For this review, take the finished solid that the model builds, in its own axes (mm). Face numbers are marked on the shaded views. A direction names the side the tool comes from. Round coordinates to 2 decimals unless told otherwise and drop trailing zeros. Write each loop counter-clockwise with the first axis right and the second up, starting at its lowest first coordinate (ties: lowest second). Pieces come first, ordered by that corner, then holes. Notation, with made-up numbers: (-12, -27.5) -> (-5, -27.5) arc R6 ccw to (-5, -23.5) -> close; hole circle Ø7 at (8.5, -27.75). An arc over 180 degrees is marked (long way). Answer in a Markdown table with one row per item.
from build123d import *

# Parameters (mm, degrees)
F0_R           = 14
F1_DEPTH       = 40
F4_D           = 11
F4_CBORE_D     = 18
F4_CBORE_DEPTH = 7.3


with BuildPart() as f1:
    # F0 (on Front) → F1 (new body)
    with BuildSketch(Plane.XZ):
        with BuildLine():
            Line((-31.928091, 15), (-31.928091, 7.7))
            Line((-31.928091, 7.7), (-31.928091, 0))
            Line((-31.928091, 0), (78.071909, 0))
            Line((78.071909, 0), (78.071909, 7.7))
            Line((78.071909, 7.7), (78.071909, 15))
            Line((78.071909, 15), (48.071909, 15))
            Line((48.071909, 15), (48.071909, 27.340618))
            Line((48.071909, 27.340618), (48.071909, 40))
            ThreePointArc((48.071909, 40), (23.071909, 65), (-1.928091, 40))
            Line((-1.928091, 40), (-1.928091, 27.340618))
            Line((-1.928091, 27.340618), (-1.928091, 15))
            Line((-1.928091, 15), (-31.928091, 15))
        make_face()
        with Locations((23.071909, 40)):
            Circle(F0_R, mode=Mode.SUBTRACT)
    extrude(amount=F1_DEPTH)

    # F4 (through all)
    with Locations(Plane.XY.offset(15)):
        with Locations((-16.928091, -20), (63.071909, -20)):
            CounterBoreHole(F4_D / 2, F4_CBORE_D / 2, F4_CBORE_DEPTH)


solid = f1.part
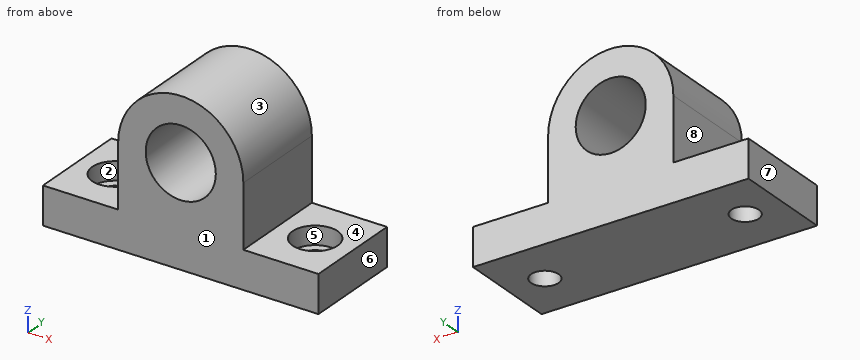
1) Clearance check with flat-ended pins moving along their axes: pin 1 Ø20 at (x, y) = (-16, -16.5) entering from +Z; pin 2 Ø3 at (x, y) = (46.5, -30.5) entering from +Z; pin 3 Ø8 at (y, z) = (-10.5, 54) entering from -X. State where each tip first meets the part, or that it passes through.
Solved:
| item | result |
|---|---|
| pin 1 | z = 15 |
| pin 2 | z = 52.01 |
| pin 3 | x = 0.16 |
2) Consider section C-C on y = -35.5. State the section outline as (x, z) points, then the cut area to 3 significant figures.
Solved:
| item | result |
|---|---|
| outline | (-31.93, 0) -> (78.07, 0) -> (78.07, 15) -> (48.07, 15) -> (48.07, 40) arc R25 ccw to (-1.93, 40) -> (-1.93, 15) -> (-31.93, 15) -> close; hole circle Ø28 at (23.07, 40) |
| area | 3,270 mm² |
3) For the marked faces 4, 5, 6, 7 and 8, list the 3-axis set-ups (+Z, -Z, +X, -X, +Y, -Y) from which the entire face can be reached by the end or side of a thin tool; tool diameter is ignored.
Solved:
| item | result |
|---|---|
| face 4 | +Z, +X, +Y, -Y |
| face 5 | +Z |
| face 6 | +Z, -Z, +X, +Y, -Y |
| face 7 | +Z, -Z, -X, +Y, -Y |
| face 8 | +Z, -X, +Y, -Y |
4) Consider section B-B on z = 11. State the section outline as (x, y) points.
Solved:
| item | result |
|---|---|
| outline | (-31.93, -40) -> (78.07, -40) -> (78.07, 0) -> (-31.93, 0) -> close; hole circle Ø18 at (-16.93, -20); hole circle Ø18 at (63.07, -20) |
5) Mouldability with a two-part tool opening along X and no side actions: class the marked faces 1, 2 and 3 as pulls with the +X half, pulls with the -X half, needs draft (parallel to the pull), parting line crosses it, or undercut.
Solved:
| item | result |
|---|---|
| face 1 | needs draft |
| face 2 | undercut |
| face 3 | parting line crosses it |
6) Consider section D-D on x = 29. State the section outline as (y, z) points.
Solved:
| item | result |
|---|---|
| outline | (-40, 0) -> (0, 0) -> (0, 27.32) -> (-40, 27.32) -> close; (-40, 52.68) -> (0, 52.68) -> (0, 64.29) -> (-40, 64.29) -> close |
7) For line 1 (X direction, y = -26.5, z = 47.5); line 2 (X direction, y = -13, z = 36); line 3 (X direction, y = -14, z = 19), list the stretches that pass through material, from the lowest coordinate up. Write a range as [from, to].
Solved:
| item | result |
|---|---|
| line 1 | [-0.78, 11.25], [34.89, 46.92] |
| line 2 | [-1.93, 9.66], [36.49, 48.07] |
| line 3 | [-1.93, 48.07] |
8) Consider section A-A on y = -20. State the section outline as (x, z) points, then the cut area to 3 significant figures.
Solved:
| item | result |
|---|---|
| outline | (-31.93, 0) -> (-22.43, 0) -> (-22.43, 7.7) -> (-25.93, 7.7) -> (-25.93, 15) -> (-31.93, 15) -> close; (-11.43, 0) -> (57.57, 0) -> (57.57, 7.7) -> (54.07, 7.7) -> (54.07, 15) -> (48.07, 15) -> (48.07, 40) arc R25 ccw to (-1.93, 40) -> (-1.93, 15) -> (-7.93, 15) -> (-7.93, 7.7) -> (-11.43, 7.7) -> close; (68.57, 0) -> (78.07, 0) -> (78.07, 15) -> (72.07, 15) -> (72.07, 7.7) -> (68.57, 7.7) -> close; hole circle Ø28 at (23.07, 40) |
| area | 2,830 mm² |
